```python
from build123d import *

# Parameters (mm, degrees)
HEAD_BOSS_EXTRUDE1_DEPTH   = 5.4
SKETCH11_R                 = 2.5
LENGTH_BOSS_EXTRUDE2_DEPTH = 40


with BuildPart() as part:
    # Sketch8 → head-Boss-Extrude1 (new body)
    with BuildSketch(Plane.XY):
        Polygon((0, 4.618802154), (-4, 2.309401077), (-4, -2.309401077), (0, -4.618802154), (4, -2.309401077), (4, 2.309401077), align=None)
    extrude(amount=HEAD_BOSS_EXTRUDE1_DEPTH)

    # Sketch9 → k'-Cut-Revolve1 (revolve, cut)
    with BuildSketch(Plane(origin=(0, 0, 0), x_dir=(0, 0, -1), z_dir=(1, 0, 0))):
        with BuildLine():
            Line((-5.4, 4.618802154), (-5.4, 4))
            ThreePointArc((-5.4, 4), (-4.524086001, 4.460011199), (-3.547550763, 4.618802154))
            Line((-3.547550763, 4.618802154), (-5.4, 4.618802154))
        make_face()
    revolve(axis=Axis((0, 0, 0), (0, 0, 1)), mode=Mode.SUBTRACT)

    # Sketch10 → flange-Revolve1 (revolve)
    with BuildSketch(Plane(origin=(0, 0, 0), x_dir=(0, 0, -1), z_dir=(1, 0, 0))):
        with BuildLine():
            Line((-1, 5.793028555), (-2.535564434, 2.5))
            Line((-2.535564434, 2.5), (0, 2.5))
            Line((0, 2.5), (0, 4.9))
            ThreePointArc((0, 4.9), (-0.025077882, 5.349305019), (-0.1, 5.793028555))
            ThreePointArc((-0.1, 5.793028555), (-0.55, 5.9), (-1, 5.793028555))
        make_face()
    revolve(axis=Axis((0, 0, 0), (0, 0, 1)))

    # Sketch11 → length-Boss-Extrude2 (add)
    with BuildSketch(Plane.XY):
        Circle(SKETCH11_R)
    extrude(amount=-LENGTH_BOSS_EXTRUDE2_DEPTH)

    # Sketch12 → thread-Cut-Revolve3 (revolve, cut)
    with BuildSketch(Plane(origin=(0, 0, 0), x_dir=(0, 0, -1), z_dir=(1, 0, 0)), mode=Mode.PRIVATE) as thread_cut_revolve3_sk:
        Polygon((1.6, 2.24), (0, 2.24), (0, 2.5), (2.4, 2.5), align=None)
    revolve(thread_cut_revolve3_sk.sketch.rotate(Axis((0, 0, 0), (0, 0, -1)), 90), axis=Axis((0, 0, 0), (0, 0, -1)), mode=Mode.SUBTRACT)

    # Sketch13 → chamfer-Cut-Revolve4 (revolve, cut)
    with BuildSketch(Plane(origin=(0, 0, 0), x_dir=(0, 0, -1), z_dir=(1, 0, 0))):
        Polygon((40, 2.0095), (40, 2.5), (39.415444863, 2.5), align=None)
    revolve(axis=Axis((0, 0, -40), (0, 0, 1)), mode=Mode.SUBTRACT)

    # Sketch15 → coarse-fillet-Revolve2 (revolve)
    with BuildSketch(Plane(origin=(0, 0, 0), x_dir=(0, 0, -1), z_dir=(1, 0, 0)), mode=Mode.PRIVATE) as coarse_fillet_revolve2_sk:
        with BuildLine():
            Line((0, 2.24), (1.4, 2.24))
            ThreePointArc((1.4, 2.24), (0.77257354, 2.31741069), (0.182777402, 2.545))
            ThreePointArc((0.182777402, 2.545), (0.049192715, 2.672213204), (0, 2.85))
            Line((0, 2.85), (0, 2.24))
        make_face()
    revolve(coarse_fillet_revolve2_sk.sketch.rotate(Axis((0, 0, -40), (0, 0, 1)), 90), axis=Axis((0, 0, -40), (0, 0, 1)))


solid = part.part
```
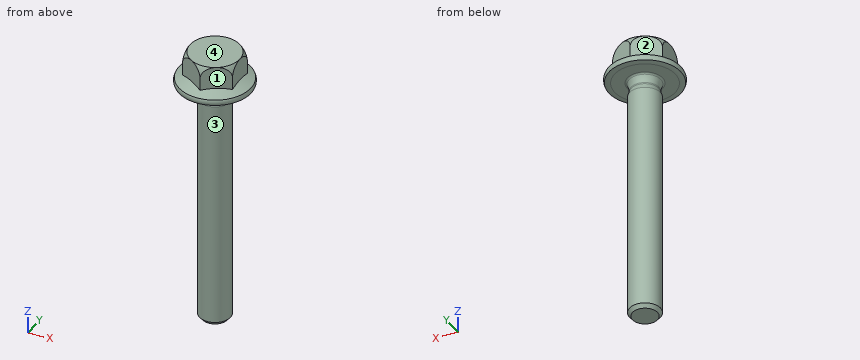
The model under review builds one solid part; all positions refer to its coordinate system, in mm. Face numbers are marked on the shaded views. A direction names the side the tool comes from. Give positions to 0.01 mm unless a question says otherwise; leave off trailing zeros. Write each loop counter-clockwise with the first axis right and the second up, starting at its lowest first coordinate (ties: lowest second). Pieces come first, ordered by that corner, then holes. Notation, with made-up numbers: (86.25, 46) -> (114.25, 46) arc R27 cw to (114.25, 69) -> close; hole circle Ø4 at (59, 82.25). An arc over 180 degrees is marked (long way). Put each result on its own line as item: value.
(1) For pin 1 Ø3 at (y, z) = (1.5, -19.5) entering from +X; pin 2 Ø1.5 at (x, z) = (-3, -15.5) entering from +Y; pin 3 Ø4 at (x, y) = (1, 4) entering from -Z, all flat-tipped, find the tip position at first contact; note any pin that passes through.
Results are:
pin 1: x = 2.5
pin 2: y = 1.09
pin 3: z = -39.86
(2) We need section A-A, the plane z = -18. Give the boundary of the cut face in (x, y).
Results are:
outline: circle Ø5 at (0, 0)
(3) Tool access review of the marked faces 1, 2, 3 and 4: name each direction out of +Z, -Z, +X, -X, +Y, -Y from which nothing blocks a thin tool from reaching the whole face with its end or side.
Results are:
face 1: +Z, +X, -Y
face 2: +Z, -X, +Y
face 3: -Z
face 4: +Z, +X, -X, +Y, -Y
(4) To check wall thickness, follow probe 1 along Z at (x, y) = (1, 3); probe 2 along Z at (x, y) = (4.75, 1.75); probe 3 along Y at (x, z) = (1.5, -20). State the ranges of each line that lie inside material, in increasing order. Write a range as from..to.
Results are:
probe 1: 0..5.4
probe 2: 0..1.34
probe 3: -2..2
